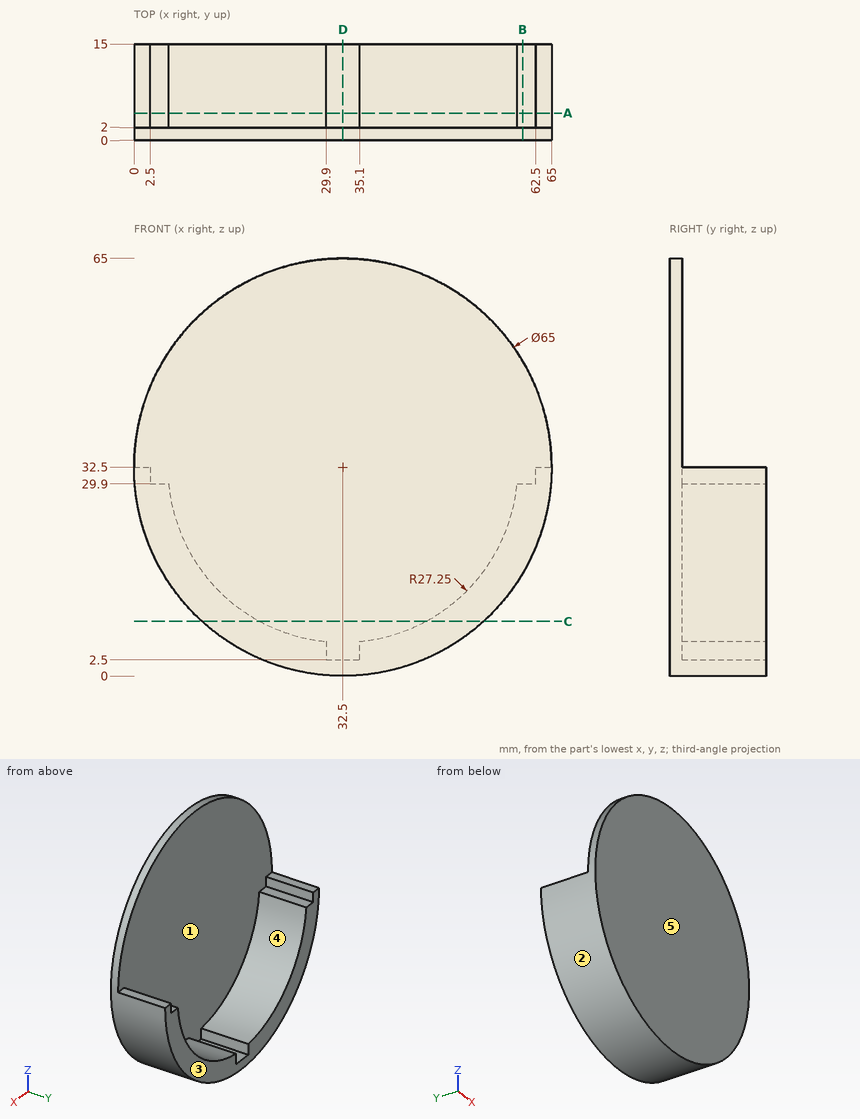
The drawing under review shows one solid part. Ordinate dimensions are in mm from its lowest x, y, z. A direction names the side the tool comes from. Round coordinates to 2 decimals unless told otherwise and drop trailing zeros. Loops run counter-clockwise (first coordinate to the right, second up) from the corner with the lowest first, then second, coordinate; pieces in that order, holes last. Notation, with made-up numbers: (10.5, 26) - (30.5, 26) arc R21 cw to (30.5, 33) - close; hole circle Ø4 at (-11.5, 53). An arc over 180 degrees is marked (long way). Use one line per item in the form item = value.
Item 1: Tool access review of the marked faces 4 and 5: name each direction out of +Z, -Z, +X, -X, +Y, -Y from which nothing blocks a thin tool from reaching the whole face with its end or side.
Answers:
face_4 = +Z, +Y
face_5 = +Z, -Z, +X, -X, -Y
Item 2: Clearance check with flat-ended pins moving along their axes: P1, Ø5.5, axis at x = 33, y = 6.5, coming from the +Z side; P2, Ø1.4, axis at x = 4.5, y = 7.5, coming from the +Z side; P3, Ø2, axis at x = 23.5, z = 58, coming from the +Y side. State where each tip first meets the part, or that it passes through.
Answers:
P1 = 5.44
P2 = 29.9
P3 = 2
Item 3: Consider section A-A on y = 4.25. Write out the cut boundary in (x, z), then the cut area to 3 significant figures.
Answers:
outline = (0, 32.5) arc R32.5 ccw to (65, 32.5) - (62.5, 32.5) - (62.5, 29.9) - (59.63, 29.9) arc R27.25 cw to (35.1, 5.37) - (35.1, 2.5) - (29.9, 2.5) - (29.9, 5.37) arc R27.25 cw to (5.37, 29.9) - (2.5, 29.9) - (2.5, 32.5) - close
area = 464 mm^2
Item 4: Consider section B-B on x = 60.5. Write out the cut boundary in (y, z).
Answers:
outline = (0, 16) - (15, 16) - (15, 29.9) - (2, 29.9) - (2, 49) - (0, 49) - close
Item 5: Consider section D-D on x = 32.5. Write out the cut boundary in (y, z).
Answers:
outline = (0, 0) - (15, 0) - (15, 2.5) - (2, 2.5) - (2, 65) - (0, 65) - close
Item 6: Mouldability with a two-part tool opening along X and no side actions: class the marked faces 1, 2 and 3 as +X half, -X half, draft (parallel to the pull), parting line (faces both ways), or undercut.
Answers:
face_1 = undercut
face_2 = parting line
face_3 = draft
Item 7: Consider section C-C on z = 8.5. Write out the cut boundary in (x, y).
Answers:
outline = (10.59, 0) - (54.41, 0) - (54.41, 15) - (45.41, 15) - (45.41, 2) - (19.59, 2) - (19.59, 15) - (10.59, 15) - close
Item 8: For line 1 (Y direction, x = 38.5, z = 58.5); line 2 (X direction, y = 12.75, z = 27); line 3 (Z direction, x = 33, y = 13), list the stretches that pass through material, from the lowest coordinate up.
Answers:
line_1 = 0 to 2
line_2 = 0.47 to 5.81, 59.19 to 64.53
line_3 = 0 to 2.5
